Part model, mm, in its own coordinate system. A direction names the side the tool comes from. Round coordinates to 2 decimals unless told otherwise and drop trailing zeros. Order: outer loops, then holes, each group sorted by start corner. A loop starts at its lowest first (then second) coordinate and runs counter-clockwise, first axis right, second up. Notation, with made-up numbers: M -9,38 L 39,38 A20 ccw 39,51 Z; hole C 68.5,24 d1. An arc over 180 degrees is marked long. One line per question, with ' | ' between items.
from build123d import *

# Parameters (mm, degrees)
ESTRUSIONE_ESTRUSIONE2_DEPTH = 55
NERVATURA1_REACH             = 177.707
SCHIZZO2_WALL_W              = 409.315984862
SCHIZZO2_WALL_H              = 4
SCHIZZO3_W                   = 84
SCHIZZO3_H                   = 104
TAGLIO_ESTRUSIONE1_DEPTH     = 30
SCHIZZO4_W                   = 74
SCHIZZO4_H                   = 14
TAGLIO_ESTRUSIONE2_DEPTH     = 33
SPECCHIA2_START              = -77
SPECCHIA2_DEPTH              = 22
SPECCHIA2_START_2            = -110
SPECCHIA2_2_OUTLINE_W        = 14
SPECCHIA2_2_OUTLINE_H        = 44
SPECCHIA2_2_DEPTH            = 33
SPECCHIA2_START_3            = -80
SPECCHIA2_3_DEPTH            = 3
SPECCHIA2_START_4            = -59
SPECCHIA2_4_DEPTH            = 4
RACCORDO1_RADIUS             = 22
RACCORDO1_LENGTH             = 14
RACCORDO3_R                  = 20
RACCORDO4_R                  = 6
TAGLIO_ESTRUSIONE3_DEPTH     = 184.760713973
SCHIZZO7_W                   = 3
SCHIZZO7_H                   = 45
TAGLIO_ESTRUSIONE4_DEPTH     = 192.397492147
RACCORDO11_RADIUS            = 22
RACCORDO11_LENGTH            = 11
RACCORDO12_R                 = 6
RACCORDO13_R                 = 16
RACCORDO15_R                 = 10
SCHIZZO8_R                   = 10
TAGLIO_ESTRUSIONE5_DEPTH     = 192.397492147
SCHIZZO9_R                   = 11.5
ESTRUSIONE_ESTRUSIONE3_DEPTH = 5
SCHIZZO10_R                  = 6
TAGLIO_ESTRUSIONE6_DEPTH     = 190.274932307
TAGLIO_ESTRUSIONE7_REACH     = 201.87
RACCORDO17_R                 = 4
RACCORDO18_START             = 75
RACCORDO18_DEPTH             = 13


with BuildPart() as part:
    # Schizzo1 → Estrusione-Estrusione2 (new body)
    with BuildSketch(Plane(origin=(0, 0, 0), x_dir=(0, 0, -1), z_dir=(1, 0, 0))):
        Polygon((0, 0), (-118, 0), (-118, 14), (-88, 14), (-88, 73), (-15, 73), (-15, 118), (-4, 118), (-4, 60), (-75, 60), (-75, 14), (0, 14), align=None)
    extrude(amount=-ESTRUSIONE_ESTRUSIONE2_DEPTH)

    # Schizzo2 wall → Nervatura1 (add, up to next)
    with BuildSketch(Plane(origin=(-55, 39, 100.5), x_dir=(0, -0.894427191, 0.4472135955), z_dir=(0, 0.4472135955, 0.894427191)), mode=Mode.PRIVATE) as nervatura1_sk1:
        with Locations((0, 2)):
            Rectangle(SCHIZZO2_WALL_W, SCHIZZO2_WALL_H)
    nervatura1_tool1 = extrude(nervatura1_sk1.sketch, amount=-NERVATURA1_REACH, mode=Mode.PRIVATE) - part.part
    add(nervatura1_tool1.solids().sort_by_distance((-55, 39, 100.5))[0])

    # Schizzo3 → Taglio-Estrusione1 (cut)
    with BuildSketch(Plane(origin=(0, 0, 0), x_dir=(0, 0, -1), z_dir=(1, 0, 0))):
        with Locations((-46, 66)):
            Rectangle(SCHIZZO3_W, SCHIZZO3_H)
    extrude(amount=-TAGLIO_ESTRUSIONE1_DEPTH, mode=Mode.SUBTRACT)

    # Schizzo4 → Taglio-Estrusione2 (cut)
    with BuildSketch(Plane(origin=(0, 0, 0), x_dir=(0, 0, -1), z_dir=(1, 0, 0))):
        with Locations((-37, 7)):
            Rectangle(SCHIZZO4_W, SCHIZZO4_H)
    extrude(amount=-TAGLIO_ESTRUSIONE2_DEPTH, mode=Mode.SUBTRACT)

    # Specchia2: read off the stored shape, not the designer's step
    # Specchia2 outline → Specchia2 (add)
    with BuildSketch(Plane.YZ.offset(SPECCHIA2_START)):
        Polygon((0, 0), (14, 0), (14, 75), (60, 75), (60, 4), (118, 4), (118, 15), (73, 15), (73, 88), (14, 88), (14, 118), (0, 118), align=None)
    extrude(amount=SPECCHIA2_DEPTH)

    # Specchia2 2 outline → Specchia2 2 (add)
    with BuildSketch(Plane.YZ.offset(SPECCHIA2_START_2)):
        with Locations((7, 96)):
            Rectangle(SPECCHIA2_2_OUTLINE_W, SPECCHIA2_2_OUTLINE_H)
    extrude(amount=SPECCHIA2_2_DEPTH)

    # Specchia2 3 outline → Specchia2 3 (add)
    with BuildSketch(Plane.YZ.offset(SPECCHIA2_START_3)):
        Polygon((14, 88), (14, 75), (60, 75), (60, 4), (118, 4), (118, 15), (73, 15), (73, 88), align=None)
    extrude(amount=SPECCHIA2_3_DEPTH)

    # Specchia2 4 outline → Specchia2 4 (add)
    with BuildSketch(Plane.YZ.offset(SPECCHIA2_START_4)):
        Polygon((14, 113), (14, 88), (64, 88), align=None)
    extrude(amount=SPECCHIA2_4_DEPTH)

    # Raccordo1: full round fillet: the end face becomes a half cylinder, R = half its width
    raccordo1_face = Plane((-55, 7, 0), x_dir=(0, -1, 0), z_dir=(0, 0, -1))  # on the end face: x along it, z out of the body
    raccordo1_slab = raccordo1_face.offset(-RACCORDO1_RADIUS / 2) * Box(RACCORDO1_LENGTH, 2 * RACCORDO1_RADIUS, RACCORDO1_RADIUS, mode=Mode.PRIVATE)  # the body's end, R deep
    raccordo1_round = Plane((-55, 7, 22), x_dir=(0, 0, -1), z_dir=(0, -1, 0)) * Cylinder(RACCORDO1_RADIUS, RACCORDO1_LENGTH, mode=Mode.PRIVATE)  # its axis R under the face
    add(raccordo1_slab - raccordo1_round, mode=Mode.SUBTRACT)

    # Raccordo3
    raccordo3_edges = [part.edges().sort_by_distance(p)[0] for p in [
        (-33, 7, 74),
        (-77, 7, 74),
    ]]
    fillet(raccordo3_edges, radius=RACCORDO3_R)

    # Raccordo4
    raccordo4_edges = [part.edges().sort_by_distance(p)[0] for p in [
        (0, 7, 74),
        (-110, 7, 118),
        (0, 7, 118),
        (-110, 7, 74),
    ]]
    fillet(raccordo4_edges, radius=RACCORDO4_R)

    # Schizzo6 → Taglio-Estrusione3 (cut, through all)
    with BuildSketch(Plane.XY.offset(88)):
        Polygon((-33, 73), (-30, 14), (-30, 73), align=None)
        Polygon((-80, 14), (-80, 73), (-77, 73), align=None)
    extrude(amount=-TAGLIO_ESTRUSIONE3_DEPTH, mode=Mode.SUBTRACT)

    # Schizzo7 → Taglio-Estrusione4 (cut, through all)
    with BuildSketch(Plane.XY.offset(15)):
        with Locations((-31.5, 95.5)):
            Rectangle(SCHIZZO7_W, SCHIZZO7_H)
        with Locations((-78.5, 95.5)):
            Rectangle(SCHIZZO7_W, SCHIZZO7_H)
    extrude(amount=-TAGLIO_ESTRUSIONE4_DEPTH, mode=Mode.SUBTRACT)

    # Raccordo11: full round fillet: the end face becomes a half cylinder, R = half its width
    raccordo11_face = Plane((-55, 118, 9.5), x_dir=(0, 0, -1), z_dir=(0, 1, 0))  # on the end face: x along it, z out of the body
    raccordo11_slab = raccordo11_face.offset(-RACCORDO11_RADIUS / 2) * Box(RACCORDO11_LENGTH, 2 * RACCORDO11_RADIUS, RACCORDO11_RADIUS, mode=Mode.PRIVATE)  # the body's end, R deep
    raccordo11_round = Plane((-55, 96, 9.5), x_dir=(0, 1, 0), z_dir=(0, 0, -1)) * Cylinder(RACCORDO11_RADIUS, RACCORDO11_LENGTH, mode=Mode.PRIVATE)  # its axis R under the face
    add(raccordo11_slab - raccordo11_round, mode=Mode.SUBTRACT)

    # Raccordo12
    raccordo12_edges = [part.edges().sort_by_distance(p)[0] for p in [
        (-55, 73, 15),
        (-55, 73, 88),
    ]]
    fillet(raccordo12_edges, radius=RACCORDO12_R)

    # Raccordo13
    # the kernel refuses this fillet: 16 mm, written as the material it adds along each edge
    with BuildSketch(Plane(origin=(-59, 64, 88), x_dir=(7.107647619401389e-15, 0.9999992149494827, -0.0012530364791798036), z_dir=(1, 0, 0))) as raccordo13_piece_1:
        with BuildLine():
            CenterArc((3.78664302, 15.989963147), RACCORDO13_R, 243.506742544, 24.463710432)
            Line((-3.350836892, 1.670173327), (-4.064584883, 0.238194345))
            Line((-4.064584883, 0.238194345), (-0.713747991, -1.431978982))
            Line((-0.713747991, -1.431978982), (0.002004858, -1.599998744))
            ThreePointArc((0.002004858, -1.599998744), (3.002002503, -1.596239634), (3.163341295, -1.598996315))
            Line((3.163341295, -1.598996315), (3.220005088, 0))
        make_face()
    extrude(amount=8)

    # Raccordo15
    # the kernel refuses this fillet: 10 mm, written as the material it adds along each edge
    with BuildSketch(Plane(origin=(-51, 14, 113), x_dir=(0, 0, 1), z_dir=(-1, 0, 0))) as raccordo15_piece_1:
        with BuildLine():
            CenterArc((6.217538244, 9.925603288), RACCORDO15_R, 206.565051177, 56.441617235)
            Line((-2.726733666, 5.453467333), (-2.905619105, 5.364024614))
            Line((-2.905619105, 5.364024614), (-0.178885438, -0.089442719))
            Line((-0.178885438, -0.089442719), (0, -0.2))
            ThreePointArc((0, -0.2), (2.5, -0.2), (4.975649235, -0.198512066))
            Line((4.975649235, -0.198512066), (5, 0))
        make_face()
    extrude(amount=8)

    # Schizzo8 → Taglio-Estrusione5 (cut, through all)
    with BuildSketch(Plane.XY.offset(15)):
        with Locations((-55, 96)):
            Circle(SCHIZZO8_R)
    extrude(amount=-TAGLIO_ESTRUSIONE5_DEPTH, mode=Mode.SUBTRACT)

    # Schizzo9 → Estrusione-Estrusione3 (add)
    with BuildSketch(Plane(origin=(0, 14, 0), x_dir=(1, 0, 0), z_dir=(0, 1, 0))):
        with Locations(Location((-90, -100.149267902, 0), (0, 0, 270))):
            Circle(SCHIZZO9_R)
        with Locations(Location((-20, -100.149267902, 0), (0, 0, 270))):
            Circle(SCHIZZO9_R)
    extrude(amount=ESTRUSIONE_ESTRUSIONE3_DEPTH)

    # Schizzo10 → Taglio-Estrusione6 (cut, through all)
    with BuildSketch(Plane(origin=(0, 19, 0), x_dir=(1, 0, 0), z_dir=(0, 1, 0))):
        with Locations(Location((-90, -100.149267902, 0), (0, 0, 270))):
            Circle(SCHIZZO10_R)
        with Locations(Location((-20, -100.149267902, 0), (0, 0, 270))):
            Circle(SCHIZZO10_R)
    extrude(amount=-TAGLIO_ESTRUSIONE6_DEPTH, mode=Mode.SUBTRACT)

    # Schizzo11 → Taglio-Estrusione7 (cut, up to next)
    with BuildSketch(Plane.XZ, mode=Mode.PRIVATE) as taglio_estrusione7_sk1:
        with BuildLine():
            Line((-65, 22), (-65, 42))
            ThreePointArc((-65, 42), (-55, 52), (-45, 42))
            Line((-45, 42), (-45, 22))
            ThreePointArc((-45, 22), (-55, 12), (-65, 22))
        make_face()
    taglio_estrusione7_tool1 = extrude(taglio_estrusione7_sk1.sketch, amount=-TAGLIO_ESTRUSIONE7_REACH, mode=Mode.PRIVATE) & part.part
    add(taglio_estrusione7_tool1.solids().sort_by_distance((-55, 0, 32))[0], mode=Mode.SUBTRACT)

    # Raccordo17
    raccordo17_edges = [part.edges().sort_by_distance(p)[0] for p in [
        (-90, 14, 88.649267902),
        (-20, 14, 88.649267902),
    ]]
    fillet(raccordo17_edges, radius=RACCORDO17_R)

    # Raccordo18: read off the stored shape, not the designer's step
    # Raccordo18 outline → Raccordo18 (add)
    with BuildSketch(Plane.XY.offset(RACCORDO18_START)):
        with BuildLine():
            Line((-80, 14), (-79.710408023, 19.695308884))
            ThreePointArc((-79.710408023, 19.695308884), (-81.56915401, 15.650968689), (-85.702666639, 14))
            Line((-85.702666639, 14), (-80, 14))
        make_face()
        with BuildLine():
            Line((-30.289591977, 19.695308884), (-30, 14))
            Line((-30, 14), (-24.297333361, 14))
            ThreePointArc((-24.297333361, 14), (-28.43084599, 15.650968689), (-30.289591977, 19.695308884))
        make_face()
    extrude(amount=RACCORDO18_DEPTH)


solid = part.part
1) Saw through at B-B (z = 61). List the corners of the cut face in (x, y) (3 decimals), plus the area to 3 significant figures.
The answers:
outline: M -78.265,0 L -31.735,0 L -31.735,14 L -78.265,14 Z; M -77.661,60 L -32.339,60 L -33,73 L -77,73 Z | area: 1,230 mm²
2) Probe line 1 (Y direction, x = -55, z = 9); line 2 (Y direction, x = -34.5, z = 60.5); line 3 (Z direction, x = -49.5, y = 46). List the from-to ranges inside material, lowest first. Write a range as [from, to].
The answers:
line 1: y = [0, 14], [60, 86], [106, 118] | line 2: y = [0, 14], [60, 73] | line 3: z = [75, 88]
3) Saw through at D-D (y = 82). List the corners of the cut face in (x, z), plus the area to 3 significant figures.
The answers:
outline: M -77,4 L -33,4 L -33,15 L -77,15 Z | area: 484 mm²
4) Drop flat-ended pins along their axis: pin 1 (2 mm diameter, centred on x = -60.5, y = 37, fed in from +Z); pin 2 (15.5 mm diameter, centred on x = -90, z = 100.15, fed in from +Y); pin 3 (15.5 mm diameter, centred on y = 5, z = 44.5, fed in from +X). Give the stop position or say it passes through.
The answers:
pin 1: stops at z = 88 | pin 2: stops at y = 19 | pin 3: stops at x = -33
5) Saw through at A-A (x = -55). List the corners of the cut face in (y, z).
The answers:
outline: M 0,0 L 14,0 L 14,12 L 0,12 Z; M 0,52 L 14,52 L 14,75 L 60,75 L 60,4 L 86,4 L 86,15 L 79,15 A6 cw 73,21 L 73,82 A6 ccw 67.22,88 A16 cw 60.65,89.67 L 19.45,110.27 A10 cw 14,118 L 0,118 Z; M 106,4 L 118,4 L 118,15 L 106,15 Z
6) Saw through at C-C (x = -20). List the corners of the cut face in (y, z) (3 decimals).
The answers:
outline: M 0,72.735 L 14,72.735 L 14,84.649 A4 cw 18,88.649 L 19,88.649 L 19,94.149 L 0,94.149 Z; M 0,106.149 L 19,106.149 L 19,111.649 L 18,111.649 A4 cw 14,115.649 L 14,118 L 0,118 Z
7) Two-plate mould, pull along Z, no slides. Class faces 1 (the face through (-54.94, 15.8, 113.39)), 2 (the face through (-85.94, 9.63, 95.73)), 3 (the face through (-101, 7, 74)), 4 (the face through (-95, 19, 105)): released by +Z, released by -Z, zero draft, split by the parting line, or undercut.
The answers:
face 1: released by +Z | face 2: undercut | face 3: released by -Z | face 4: zero draft
8) Which spindle directions (+Z, -Z, +X, -X, +Y, -Y) get a long thin tool onto all of the face, cutting with end or side? Do faces 5 (the face through (-77, 7, 38)), 6 (the face through (-55, 7, 12)), 7 (the face through (-51, 29, 97)). Say none if no direction does.
The answers:
face 5: -Z, -X, -Y | face 6: -Y | face 7: +Z, +Y
